The model under review builds one solid part; all positions refer to its coordinate system, in mm. A direction names the side the tool comes from. Give positions to 0.01 mm unless a question says otherwise; leave off trailing zeros. Order: outer loops, then holes, each group sorted by start corner. A loop starts at its lowest first (then second) coordinate and runs counter-clockwise, first axis right, second up.
```python
from build123d import *

# Parameters (mm, degrees)
SKETCH1_R               = 9.765
SKETCH1_R_2             = 4.765
BOSS_EXTRUDE1_DEPTH     = 9.5
CHAMFER1_SIZE           = 2.54
CHAMFER1_SIZE2          = 7.62
CHAMFER2_SIZE           = 7.62
CHAMFER2_SIZE2          = 2.54
CHAMFER3_SIZE           = 7.62
CHAMFER3_SIZE2          = 2.54
CHAMFER4_SIZE           = 2.54
CHAMFER4_SIZE2          = 7.62
CUT_EXTRUDE1_DEPTH      = 32.652016129
CUT_EXTRUDE1_DEPTH_BACK = 32.652016129
CUT_EXTRUDE2_DEPTH      = 32.652016189
CUT_EXTRUDE2_DEPTH_BACK = 32.652016189
SKETCH4_W               = 9.53
SKETCH4_H               = 9.53
CUT_EXTRUDE3_DEPTH      = 32.652016189
CUT_EXTRUDE3_DEPTH_BACK = 32.652016189
SKETCH5_R               = 1.59


with BuildPart() as part:
    # Sketch1 → Boss-Extrude1 (new, symmetric)
    # profile 1 of 3: a face of its own
    with BuildSketch(Plane.XY):
        with BuildLine():
            ThreePointArc((-9.705624325, -1.075212291), (-7.275117629, 6.513669357), (0, 9.765))
            Line((0, 9.765), (-22.23, 9.765))
            Line((-22.23, 9.765), (-22.23, 4.765))
            Line((-22.23, 4.765), (-9.705624325, -1.075212291))
        make_face()
    # profile 2 of 3: a face of its own
    with BuildSketch(Plane.XY):
        Circle(SKETCH1_R)
        Circle(SKETCH1_R_2, mode=Mode.SUBTRACT)
    # profile 3 of 3: a face of its own
    with BuildSketch(Plane.XY):
        with BuildLine():
            Line((28.57, 0), (9.765, 0))
            ThreePointArc((9.765, 0), (7.866135596, -5.786115777), (2.908034147, -9.321939841))
            Line((2.908034147, -9.321939841), (28.57, -5))
            Line((28.57, -5), (28.57, 0))
        make_face()
    extrude(amount=BOSS_EXTRUDE1_DEPTH, both=True)

    # Chamfer1
    chamfer1_edges = [part.edges().sort_by_distance(p)[0] for p in [
        (-22.23, 7.265, 9.5),
    ]]
    chamfer1_side = [part.faces().sort_by_distance(p)[0] for p in [
        (-22.23, 7.265, 0),
    ]]
    chamfer(chamfer1_edges, length=CHAMFER1_SIZE, length2=CHAMFER1_SIZE2, reference=chamfer1_side[0])

    # Chamfer2
    chamfer2_edges = [part.edges().sort_by_distance(p)[0] for p in [
        (-22.23, 7.265, -9.5),
    ]]
    chamfer2_side = [part.faces().sort_by_distance(p)[0] for p in [
        (-11.115, 9.220751812, -9.5),
    ]]
    chamfer(chamfer2_edges, length=CHAMFER2_SIZE, length2=CHAMFER2_SIZE2, reference=chamfer2_side[0])

    # Chamfer3
    chamfer3_edges = [part.edges().sort_by_distance(p)[0] for p in [
        (28.57, -2.5, 9.5),
    ]]
    chamfer3_side = [part.faces().sort_by_distance(p)[0] for p in [
        (-7.305, 9.291087213, 9.5),
    ]]
    chamfer(chamfer3_edges, length=CHAMFER3_SIZE, length2=CHAMFER3_SIZE2, reference=chamfer3_side[0])

    # Chamfer4
    chamfer4_edges = [part.edges().sort_by_distance(p)[0] for p in [
        (28.57, -2.5, -9.5),
    ]]
    chamfer4_side = [part.faces().sort_by_distance(p)[0] for p in [
        (28.57, -2.5, -1.27),
    ]]
    chamfer(chamfer4_edges, length=CHAMFER4_SIZE, length2=CHAMFER4_SIZE2, reference=chamfer4_side[0])

    # Sketch3 → Cut-Extrude1 (cut, two sides: drawn at the far end of the back side and taken through both)
    with BuildSketch(Plane(origin=(0, 0, 0), x_dir=(1, 0, 0), z_dir=(0, 1, 0)).offset(-CUT_EXTRUDE1_DEPTH_BACK)):
        with BuildLine():
            Line((-3.81, 5.08), (6.35, 5.08))
            ThreePointArc((6.35, 5.08), (11.43, 0), (6.35, -5.08))
            Line((6.35, -5.08), (-3.81, -5.08))
            ThreePointArc((-3.81, -5.08), (-8.89, 0), (-3.81, 5.08))
        make_face()
    extrude(amount=CUT_EXTRUDE1_DEPTH + CUT_EXTRUDE1_DEPTH_BACK, mode=Mode.SUBTRACT)

    # Sketch4 → Cut-Extrude2 (cut, two sides: drawn at the far end of the back side and taken through both)
    with BuildSketch(Plane(origin=(0, 0, 0), x_dir=(1, 0, 0), z_dir=(0, 1, 0)).offset(-CUT_EXTRUDE2_DEPTH_BACK)):
        with Locations((-17.465, 0)):
            Rectangle(SKETCH4_W, SKETCH4_H)
        with Locations((23.805, 0)):
            Rectangle(SKETCH4_W, SKETCH4_H)
    extrude(amount=CUT_EXTRUDE2_DEPTH + CUT_EXTRUDE2_DEPTH_BACK, mode=Mode.SUBTRACT)

    # Sketch5 → Cut-Extrude3 (cut, two sides: drawn at the far end of the back side and taken through both)
    with BuildSketch(Plane.XY.offset(-CUT_EXTRUDE3_DEPTH_BACK)):
        with Locations((26.03, -2.54)):
            Circle(SKETCH5_R)
        with Locations((-19.69, 7.225)):
            Circle(SKETCH5_R)
    extrude(amount=CUT_EXTRUDE3_DEPTH + CUT_EXTRUDE3_DEPTH_BACK, mode=Mode.SUBTRACT)


solid = part.part
```
Item 1: For faces 4 (the flat face through (23, -3, -4.765)), 5 (the flat face through (17, 0, 0)), 6 (the flat face through (3, 4, 9.5)), 7 (the flat face through (28.57, -3, -6)), 8 (the flat face through (-16, 6, -4.765)), list the 3-axis set-ups (+Z, -Z, +X, -X, +Y, -Y) from which the entire face can be reached by the end or side of a thin tool; tool diameter is ignored.
Values found:
face 4: +X, +Y, -Y
face 5: +Z, -Z, +X, +Y
face 6: +Z, +X, -X, +Y, -Y
face 7: +Z, -Z, +X, +Y, -Y
face 8: -X, +Y, -Y
Item 2: Take a section at D-D (x = -19.69). Give the boundary of the cut face in (y, z) (3 decimals), and give its area (3 significant figures).
Values found:
outline: (3.581, -7.807) - (5.635, -7.807) - (5.635, -4.765) - (3.581, -4.765) - close; (3.581, 4.765) - (5.635, 4.765) - (5.635, 7.807) - (3.581, 7.807) - close; (8.815, -7.807) - (9.765, -7.807) - (9.765, -4.765) - (8.815, -4.765) - close; (8.815, 4.765) - (9.765, 4.765) - (9.765, 7.807) - (8.815, 7.807) - close
area: 18.3 mm2
Item 3: Take a section at C-C (y = -8). Give the boundary of the cut face in (x, z).
Values found:
outline: (-5.6, -9.5) - (10.76, -9.5) - (10.76, -2.53) arc R5.08 cw to (6.35, -5.08) - (-3.81, -5.08) arc R5.08 cw to (-5.6, -4.75) - close; (-5.6, 4.75) arc R5.08 cw to (-3.81, 5.08) - (6.35, 5.08) arc R5.08 cw to (10.76, 2.53) - (10.76, 9.5) - (-5.6, 9.5) - close
Item 4: Draft analysis for pull direction X (two halves, no side actions). For faces 1 (the flat face through (28.57, -3, 6)), 2 (the flat face through (23, -3, 4.765)), 3 (the cylindrical face through (-18.173, 7.703, -6.179)), state which applies: released by +X, released by -X, zero draft, split by the parting line, or undercut.
Values found:
face 1: released by +X
face 2: zero draft
face 3: undercut
Item 5: Take a section at B-B (z = -1.75). Give the boundary of the cut face in (x, y) (3 decimals).
Values found:
outline: (-12.7, 0.321) - (-9.706, -1.075) arc R9.765 ccw to (-8.579, -4.664) - (-8.579, 9.765) - (-12.7, 9.765) - close; (11.119, -7.939) - (19.04, -6.605) - (19.04, 0) - (11.119, 0) - close
Item 6: For line 1 (X direction, y = -2.54, z = 5.6); line 2 (Z direction, x = -14, y = 3.5) (3 decimals); line 3 (Y direction, x = 3.5, z = -7), list the stretches that pass through material, from the lowest coordinate up.
Values found:
line 1: x = -9.43 to -4.03, 4.03 to 24.44, 27.62 to 28.57
line 2: z = -9.5 to -4.765, 4.765 to 9.5
line 3: y = -9.22 to -3.23, 3.23 to 9.12
Item 7: Take a section at A-A (x = -6.5). Give the boundary of the cut face in (y, z) (3 decimals), and give its area (3 significant figures).
Values found:
outline: (-7.287, -9.5) - (9.765, -9.5) - (9.765, -4.309) - (-7.287, -4.309) - close; (-7.287, 4.309) - (9.765, 4.309) - (9.765, 9.5) - (-7.287, 9.5) - close
area: 177 mm2
Item 8: Clearance check with flat-ended pins moving along their axes: pin 1 Ø6 at (x, y) = (22, 5.5) entering from -Z (1 decimal); pin 2 Ø1.5 at (y, z) = (-7, 1) entering from +X; pin 3 Ø6 at (x, z) = (-11.5, 7) entering from -Y; pin 4 Ø3 at (x, y) = (-19, 5.5) entering from -Z. State where each tip first meets the part, or that it passes through.
Values found:
pin 1: passes through
pin 2: stops at x = 19.04
pin 3: stops at y = -4.81
pin 4: stops at z = -8.54
